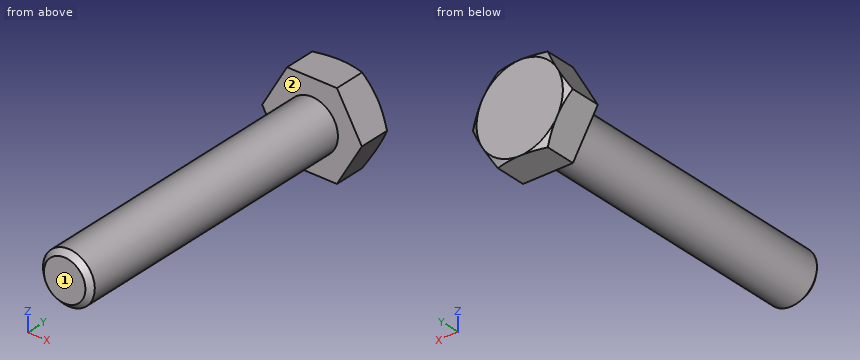
```python
from build123d import *

# Parameters (mm, degrees)
ESQUISSE2_R             = 3
BASE_EXTRUSION_DEPTH    = 35
CHANFREIN1_SIZE         = 0.6
ESQUISSE6_OUTSIDE_W     = 24.908
ESQUISSE6_OUTSIDE_H     = 24.908
ENL_V_MAT_EXTRU_1_DEPTH = 4


with BuildPart() as part:
    # Esquisse2 → Base-Extrusion (new body)
    with BuildSketch(Plane(origin=(0, 0, 0), x_dir=(1, 0, 0), z_dir=(0, 1, 0))):
        with Locations(Location((0, 0, 0), (0, 0, 270))):  # turned: the seam where the file's is
            Circle(ESQUISSE2_R)
    extrude(amount=-BASE_EXTRUSION_DEPTH)

    # Chanfrein1
    chanfrein1_edges = [part.edges().sort_by_distance(p)[0] for p in [
        (0, -35, -3),
    ]]
    chamfer(chanfrein1_edges, length=CHANFREIN1_SIZE)

    # Esquisse5 → Boss.-Révol.1 (revolve)
    with BuildSketch(Plane.XY, mode=Mode.PRIVATE) as boss_r_vol_1_sk:
        Polygon((0, 0), (7.071067812, 0), (7.071067812, 2.804268441), (5, 4), (0, 4), align=None)
    revolve(boss_r_vol_1_sk.sketch.rotate(Axis((0, 4, 0), (0, -1, 0)), 90), axis=Axis((0, 4, 0), (0, -1, 0)))  # turned: the seam where the file's is

    # Esquisse6 outside → Enlèv. mat.-Extru.1 (cut)
    with BuildSketch(Plane.XZ):
        Rectangle(ESQUISSE6_OUTSIDE_W, ESQUISSE6_OUTSIDE_H)
        Polygon((-2.886751346, -5), (2.886751346, -5), (5.773502692, 0), (2.886751346, 5), (-2.886751346, 5), (-5.773502692, 0), align=None, mode=Mode.SUBTRACT)
    extrude(amount=-ENL_V_MAT_EXTRU_1_DEPTH, mode=Mode.SUBTRACT)


solid = part.part
```
Verification items for the finished model (mm, model axes). Face numbers are marked on the shaded views. A direction names the side the tool comes from. Coordinates: 2 decimals unless noted, no trailing zeros. Loops run counter-clockwise (first coordinate to the right, second up) from the corner with the lowest first, then second, coordinate; pieces in that order, holes last. Notation, with made-up numbers: (87.5, -17) - (115.5, -17) arc R32 ccw to (115.5, 21) - close; hole circle Ø6 at (70, 65). An arc over 180 degrees is marked (long way). Answer as a JSON object with one key per item and string values.
(1) Scan lines: line 1 along Y through (x, z) = (-3.75, -0.75); line 2 along X through (y, z) = (-25.5, -0.25); line 3 along Z through (x, y) = (0.75, -26). Record each from-to range of solid material in increasing order.
Response:
{"line 1": "y = 0 to 4", "line 2": "x = -2.99 to 2.99", "line 3": "z = -2.9 to 2.9"}
(2) Cross-section at A-A, the plane y = -27.5. Record the boundary of the cut face in (x, z), then the cut area to 3 significant figures.
Response:
{"outline": "circle Ø6 at (0, 0)", "area": "28.3 mm²"}
(3) Access from +Z, -Z, +X, -X, +Y, -Y to the whole of each face (thin tool, end or side, straight path). Record for the marked faces 1 and 2.
Response:
{"face 1": "+Z, -Z, +X, -X, -Y", "face 2": "-Y"}
(4) Go/stop test with flat-tipped pins: pin 1 Ø2 at (y, z) = (-18.5, 1) entering from -X; pin 2 Ø4 at (y, z) = (-22.5, -2) entering from +X; pin 3 Ø3 at (x, z) = (-2.5, -2) entering from -Y; pin 4 Ø4 at (x, y) = (0.5, -4) entering from -Z. Record where each tip stops, or that it passes through.
Response:
{"pin 1": "stops at x = -3", "pin 2": "stops at x = 3", "pin 3": "stops at y = -35", "pin 4": "stops at z = -3"}
